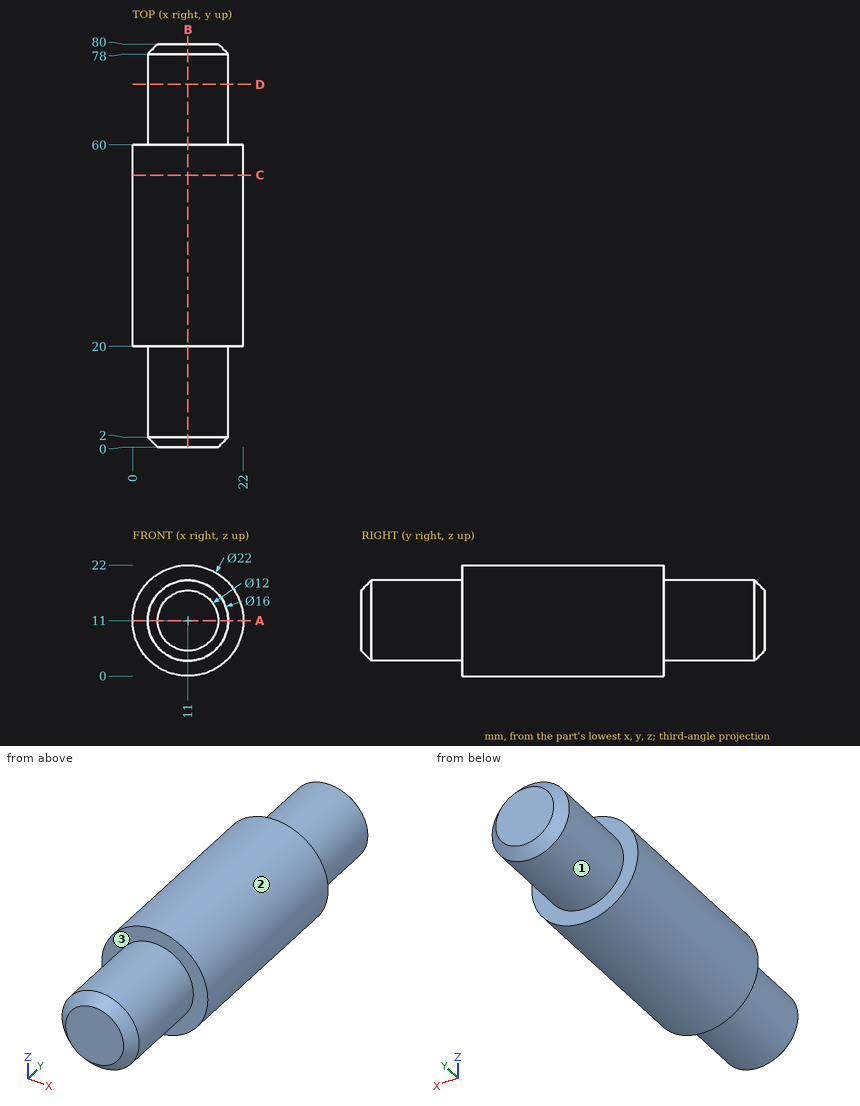
The figure shows three views and two pictorial views of one solid part (mm, origin at its lowest corner). Answer the questions. A direction names the side the tool comes from. Give positions to 0.01 mm unless a question says otherwise; leave off trailing zeros. Write each loop counter-clockwise with the first axis right and the second up, starting at its lowest first coordinate (ties: lowest second). Pieces come first, ordered by that corner, then holes. Notation, with made-up numbers: (35.5, 18.5) -> (56.5, 18.5) arc R20 cw to (56.5, 23.5) -> close; hole circle Ø7 at (14.5, 78). An arc over 180 degrees is marked (long way). Write each question's results on one line, items separated by ' | '.
1. Straight lines are drawn through the part: L1, parallel to Y at x = 19.5, z = 5.25; L2, parallel to X at y = 40.5, z = 13.75; L3, parallel to X at y = 57, z = 18.5. For each, find the intervals that lie inside material, in ascending order.
Data:
L1: 20 to 60 | L2: 0.35 to 21.65 | L3: 2.95 to 19.05
2. A tool of negligible diameter and unlimited length cuts with its end or side. For the marked faces 1, 2 and 3, from which of +Z, -Z, +X, -X, +Y, -Y can it reach the whole face along a straight path? Write none if from no direction.
Data:
face 1: +Y | face 2: +Y, -Y | face 3: -Y
3. Find section B-B on x = 11. Determine the outline of the cut face in (y, z).
Data:
outline: (0, 5) -> (2, 3) -> (20, 3) -> (20, 0) -> (60, 0) -> (60, 3) -> (78, 3) -> (80, 5) -> (80, 17) -> (78, 19) -> (60, 19) -> (60, 22) -> (20, 22) -> (20, 19) -> (2, 19) -> (0, 17) -> close
4. Find section A-A on z = 11. Determine the outline of the cut face in (x, y), and give its area (3 significant figures).
Data:
outline: (0, 20) -> (3, 20) -> (3, 2) -> (5, 0) -> (17, 0) -> (19, 2) -> (19, 20) -> (22, 20) -> (22, 60) -> (19, 60) -> (19, 78) -> (17, 80) -> (5, 80) -> (3, 78) -> (3, 60) -> (0, 60) -> close | area: 1,510 mm^2
5. Find section C-C on y = 54. Determine the outline of the cut face in (x, z).
Data:
outline: circle Ø22 at (11, 11)
6. Each of these flat-tipped pins is pushed along its axis until it touches: pin 1 Ø12 at (y, z) = (59, 19) entering from -X; pin 2 Ø1 at (x, y) = (16.5, 71) entering from +Z (3 decimals); pin 3 Ø6 at (x, y) = (2.5, 10.5) entering from +Z. Where does it stop, or does it pass through?
Data:
pin 1: x = 0.18 | pin 2: z = 17.245 | pin 3: z = 16.81
7. Find section D-D on y = 72. Determine the outline of the cut face in (x, z), and give its area (3 significant figures).
Data:
outline: circle Ø16 at (11, 11) | area: 201 mm^2
